Design review of the part built by this model. Coordinates are the model's own, in mm. A direction names the side the tool comes from. Coordinates: 2 decimals unless noted, no trailing zeros. Write each loop counter-clockwise with the first axis right and the second up, starting at its lowest first coordinate (ties: lowest second). Pieces come first, ordered by that corner, then holes. Notation, with made-up numbers: (86, 4) - (141, 4) arc R17 ccw to (141, 34) - close; hole circle Ø7 at (-25, -34.5). An arc over 180 degrees is marked (long way). Use a Markdown table: item, result.
from build123d import *

# Parameters (mm, degrees)
SKETCH1_W             = 8
SKETCH1_H             = 121
BOSS_EXTRUDE1_DEPTH   = 4
FILLET1_R             = 3
CUT_EXTRUDE1_DEPTH    = 4
F_1_0MM_DOWEL_HOLE1_D = 3
SKETCH6_R             = 0.6
CUT_EXTRUDE2_DEPTH    = 10


with BuildPart() as part:
    # Sketch1 → Boss-Extrude1 (new body)
    with BuildSketch(Plane.XY):
        Rectangle(SKETCH1_W, SKETCH1_H)
    extrude(amount=BOSS_EXTRUDE1_DEPTH)

    # Fillet1
    fillet1_edges = [part.edges().sort_by_distance(p)[0] for p in [
        (4, -60.5, 2),
        (-4, -60.5, 2),
    ]]
    fillet(fillet1_edges, radius=FILLET1_R)

    # Sketch2 → Cut-Extrude1 (cut)
    with BuildSketch(Plane.XY.offset(4)):
        Polygon((-4, 25.5), (-2, 50.5), (-2, 60.5), (-4, 60.5), align=None)
        Polygon((2, 60.5), (2, 50.5), (4, 25.5), (4, 60.5), align=None)
    extrude(amount=-CUT_EXTRUDE1_DEPTH, mode=Mode.SUBTRACT)

    # Ø1.0mm Dowel Hole1 (through all)
    with Locations(Plane.XY.offset(4)):
        with Locations((0, -56.5)):
            Hole(F_1_0MM_DOWEL_HOLE1_D / 2)

    # Sketch6 → Cut-Extrude2 (cut)
    with BuildSketch(Plane.XY.offset(4)):
        with Locations((0, -6.5)):
            Circle(SKETCH6_R)
    extrude(amount=-CUT_EXTRUDE2_DEPTH, mode=Mode.SUBTRACT)


solid = part.part
(1) Take a section at B-B on z = 2.05. Write out the cut boundary in (x, y), and give its area (3 significant figures).
Determined:
| item | result |
|---|---|
| outline | (-4, -57.5) arc R3 ccw to (-1, -60.5) - (1, -60.5) arc R3 ccw to (4, -57.5) - (4, 25.5) - (2, 50.5) - (2, 60.5) - (-2, 60.5) - (-2, 50.5) - (-4, 25.5) - close; hole circle Ø3 at (0, -56.5); hole circle Ø1.2 at (0, -6.5) |
| area | 866 mm2 |
(2) Draft analysis for pull direction X (two halves, no side actions). For faces 4 (the cylindrical face through (0, -55, 2)), 5 (the cylindrical face through (3.1, -59.64, 2.03)), 6 (the cylindrical face through (-3.14, -59.6, 2.03)), state which applies: +X half, -X half, draft (parallel to the pull), parting line (faces both ways), or undercut.
Determined:
| item | result |
|---|---|
| face 4 | undercut |
| face 5 | +X half |
| face 6 | -X half |
(3) Take a section at C-C on y = 46. Write out the cut boundary in (x, z).
Determined:
| item | result |
|---|---|
| outline | (-2.36, 0) - (2.36, 0) - (2.36, 4) - (-2.36, 4) - close |
(4) For L1, parallel to Y at x = 0, z = 2.1; L2, parallel to X at y = 52, z = 1.3; L3, parallel to X at y = 44.5, z = 3.3, list the stretches that pass through material, from the lowest coordinate up. Write a range as from..to.
Determined:
| item | result |
|---|---|
| L1 | -60.5..-58, -55..-7.1, -5.9..60.5 |
| L2 | -2..2 |
| L3 | -2.48..2.48 |
(5) Take a section at D-D on x = 3. Write out the cut boundary in (y, z).
Determined:
| item | result |
|---|---|
| outline | (-59.74, 0) - (38, 0) - (38, 4) - (-59.74, 4) - close |
(6) Take a section at A-A on y = -56.5. Write out the cut boundary in (x, z), and give its area (3 significant figures).
Determined:
| item | result |
|---|---|
| outline | (-4, 0) - (-1.5, 0) - (-1.5, 4) - (-4, 4) - close; (1.5, 0) - (4, 0) - (4, 4) - (1.5, 4) - close |
| area | 20.0 mm2 |
(7) For pin 1 (2 mm diameter, centred on y = 55, z = 2.5, fed in from -X); pin 2 (2 mm diameter, centred on y = 56, z = 2, fed in from +X); pin 3 (4 mm diameter, centred on x = 0, y = -56.5, fed in from -Z), all flat-tipped, find the tip position at first contact; note any pin that passes through.
Determined:
| item | result |
|---|---|
| pin 1 | x = -2 |
| pin 2 | x = 2 |
| pin 3 | z = 0 |
(8) Machinability: for faces 1 (the flat face through (0, 1, 0)), 2 (the flat face through (-2, 55, 2)), 3 (the flat face through (2, 56, 2)), which of the approach directions +Z, -Z, +X, -X, +Y, -Y give a long, thin tool a straight path to every point of the face, cutting with its end or side? Answer none if there is none.
Determined:
| item | result |
|---|---|
| face 1 | -Z, +X, -X, +Y, -Y |
| face 2 | +Z, -Z, -X, +Y |
| face 3 | +Z, -Z, +X, +Y |
